Model file for the job. Use its own axes, mm. Face numbers are marked on the shaded views. A direction names the side the tool comes from. Coordinates: 2 decimals unless noted, no trailing zeros. Order: outer loops, then holes, each group sorted by start corner. A loop starts at its lowest first (then second) coordinate and runs counter-clockwise, first axis right, second up. Notation, with made-up numbers: M 19.5,34 L 36.5,34 A24 ccw 36.5,52 Z; hole C 26.25,-22 d10. An arc over 180 degrees is marked long. Return JSON: item names as keys, results as strings.
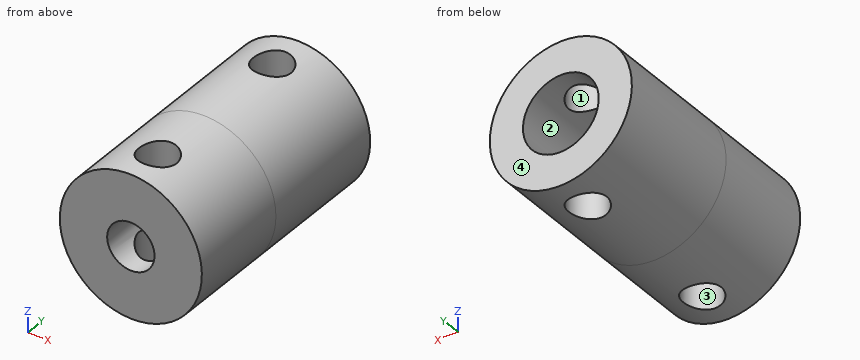
```python
from build123d import *

# Parameters (mm, degrees)
SKETCH1_R               = 7.5
SKETCH1_R_2             = 4
BOSS_EXTRUDE1_DEPTH     = 14
BOSS_EXTRUDE2_START     = 11
SKETCH2_R               = 7.5
SKETCH2_R_2             = 2.5
BOSS_EXTRUDE2_DEPTH     = 11
CUT_EXTRUDE1_DEPTH      = 18.56416807
CUT_EXTRUDE1_DEPTH_BACK = 18.56416807
SKETCH3_R               = 2


with BuildPart() as part:
    # Sketch1 → Boss-Extrude1 (new body)
    with BuildSketch(Plane(origin=(0, 0, 0), x_dir=(1, 0, 0), z_dir=(0, 1, 0))):
        with Locations(Location((0, 0, 0), (0, 0, 270))):
            Circle(SKETCH1_R)
        with Locations(Location((0, 0, 0), (0, 0, 270))):
            Circle(SKETCH1_R_2, mode=Mode.SUBTRACT)
    extrude(amount=BOSS_EXTRUDE1_DEPTH)

    # Sketch2 → Boss-Extrude2 (add)
    with BuildSketch(Plane.XZ.offset(BOSS_EXTRUDE2_START)):
        with Locations(Location((0, 0, 0), (0, 0, 270))):
            Circle(SKETCH2_R)
        with Locations(Location((0, 0, 0), (0, 0, 270))):
            Circle(SKETCH2_R_2, mode=Mode.SUBTRACT)
    extrude(amount=-BOSS_EXTRUDE2_DEPTH)

    # Sketch3 → Cut-Extrude1 (cut, two sides: drawn at the far end of the back side and taken through both)
    with BuildSketch(Plane.XY.offset(-CUT_EXTRUDE1_DEPTH_BACK)):
        with Locations((0, 10)):
            Circle(SKETCH3_R)
        with Locations((0, -7)):
            Circle(SKETCH3_R)
    extrude(amount=CUT_EXTRUDE1_DEPTH + CUT_EXTRUDE1_DEPTH_BACK, mode=Mode.SUBTRACT)


solid = part.part
```
Item 1: Drop flat-ended pins along their axis: pin 1 Ø4.5 at (x, y) = (0, -7) entering from +Z; pin 2 Ø2 at (x, y) = (5, 1.5) entering from -Z; pin 3 Ø4 at (y, z) = (-3.5, 4) entering from -X; pin 4 Ø3 at (y, z) = (-7, 4) entering from -X. Give the stop position or say it passes through.
Check result:
{"pin 1": "stops at z = 7.5", "pin 2": "stops at z = -6.34", "pin 3": "stops at x = -7.23", "pin 4": "stops at x = -7.07"}
Item 2: Pull direction X, two halves, no side cores. Call the marked faces 3 and 4: +X half, -X half, draft (parallel to the pull), parting line (faces both ways), or undercut.
Check result:
{"face 3": "undercut", "face 4": "draft"}
Item 3: Wall check: line 1 (Z direction, x = 0, y = -3.5); line 2 (Z direction, x = 0, y = 3.5). Give the ranges that are in metal, low to high.
Check result:
{"line 1": "z = -7.5 to -2.5, 2.5 to 7.5", "line 2": "z = -7.5 to -4, 4 to 7.5"}
Item 4: 3-axis set-ups, long thin cutter, end or side, ignore diameter. For the marked faces 1 and 2: which of +Z, -Z, +X, -X, +Y, -Y reach the whole face in a straight line?
Check result:
{"face 1": "+Z, -Z", "face 2": "+Y"}
Item 5: Saw through at A-A (x = 0). Write the cut outline in (y, z).
Check result:
{"outline": "M -11,-7.5 L -9,-7.5 L -9,-2.5 L -11,-2.5 Z; M -11,2.5 L -9,2.5 L -9,7.5 L -11,7.5 Z; M -5,-7.5 L 8,-7.5 L 8,-4 L 0,-4 L 0,-2.5 L -5,-2.5 Z; M -5,2.5 L 0,2.5 L 0,4 L 8,4 L 8,7.5 L -5,7.5 Z; M 12,-7.5 L 14,-7.5 L 14,-4 L 12,-4 Z; M 12,4 L 14,4 L 14,7.5 L 12,7.5 Z"}
Item 6: Saw through at D-D (y = -1). Write the cut outline in (x, z).
Check result:
{"outline": "C 0,0 d15; hole C 0,0 d5"}
Item 7: Saw through at C-C (z = 2). Write the cut outline in (x, y).
Check result:
{"outline": "M -7.23,-11 L -1.5,-11 L -1.5,-8.32 A2 cw -1.5,-5.68 L -1.5,0 L -3.46,0 L -3.46,14 L -7.23,14 Z; M 1.5,-11 L 7.23,-11 L 7.23,14 L 3.46,14 L 3.46,0 L 1.5,0 L 1.5,-5.68 A2 cw 1.5,-8.32 Z"}
Item 8: Saw through at B-B (y = 10). Write the cut outline in (x, z).
Check result:
{"outline": "M -2,-7.23 L -2,-3.46 A4 cw -2,3.46 L -2,7.23 A7.5 ccw Z; M 2,-7.23 A7.5 ccw 2,7.23 L 2,3.46 A4 cw 2,-3.46 Z"}
